Study the drawing (mm; zero at the part's minimum x, y, z) and answer. Coordinates: 2 decimals unless noted, no trailing zeros. Write each loop counter-clockwise with the first axis right and the second up, starting at its lowest first coordinate (ties: lowest second). Pieces come first, ordered by that corner, then holes. Notation, with made-up numbers: M 62.25,21.5 L 101.25,21.5 A34 ccw 101.25,54.5 Z; hole C 76.25,-21.75 d1. An arc over 180 degrees is marked long. Answer as a JSON object with one key per item and string values. Group by question number.
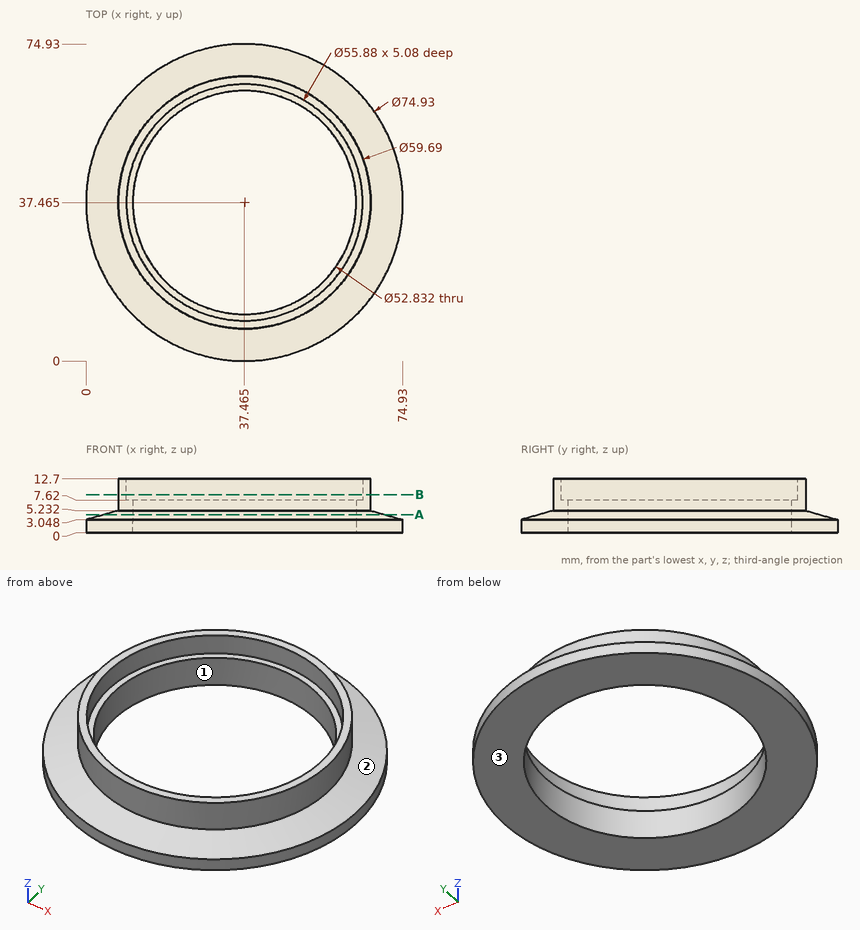
Item 1: For a pull along Y with two mould halves and no side action, classify the marked faces 1, 2 and 3 as +Y half, -Y half, draft (parallel to the pull), parting line (faces both ways), or undercut.
Item 2: Consider L1, parallel to Z at x = 23, y = 61; L2, parallel to X at y = 50.5, z = 6.5; L3, parallel to X at y = 14, z = 2.5 (1 decimal). Determine where each line is inside the solid, lowest interval first. Write a range as from..to.
Item 3: A cutting plane is placed at A-A, the plane z = 4.25. Write down the section's boundary in (x, y) (1 decimal).
Item 4: Flat-ended cylindrical pins translate along their axes: pin 1 Ø4 at (x, z) = (25.5, 2.5) entering from +Y; pin 2 Ø4 at (y, z) = (18.5, 2.5) entering from -X; pin 3 Ø1.5 at (x, z) = (52, 7) entering from -Y (1 decimal). Find the tip coordinate at first contact, or state that the pin passes through.
Item 5: A cutting plane is placed at B-B, the plane z = 9. Write down the section's boundary in (x, y) (1 decimal).
Answer:
{
 "1": {"face 1": "undercut", "face 2": "parting line", "face 3": "draft"},
 "2": {"L1": "0..7.62", "L2": "10.62..14.49, 60.44..64.31", "L3": "8.3..25.3, 49.6..66.7"},
 "3": {"outline": "C 37.5,37.5 d66.5; hole C 37.5,37.5 d52.8"},
 "4": {"pin 1": "y = 73.58", "pin 2": "x = 4.06", "pin 3": "y = 11"},
 "5": {"outline": "C 37.5,37.5 d59.7; hole C 37.5,37.5 d55.9"}
}
